Work out the finished part from the listing and answer in its coordinate system (mm). Face numbers are marked on the shaded views. A direction names the side the tool comes from. Coordinates: 2 decimals unless noted, no trailing zeros. Order: outer loops, then holes, each group sorted by start corner. A loop starts at its lowest first (then second) coordinate and runs counter-clockwise, first axis right, second up. Notation, with made-up numbers: (-8, 85) -> (1, 85) arc R4 ccw to (1, 91) -> close; hole circle Ø7 at (-15, -35). An arc over 180 degrees is marked (long way). Use one line per item in the form item = value.
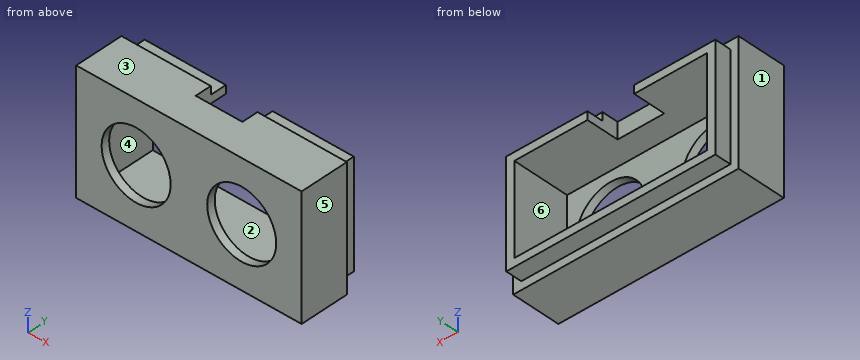
from build123d import *

# Parameters (mm, degrees)
SKETCH1_W           = 47.5
SKETCH1_H           = 22
SKETCH1_R           = 8.5
BOSS_EXTRUDE1_DEPTH = 2
SKETCH1_3_W         = 51.5
SKETCH1_3_H         = 26
SKETCH1_3_W_2       = 47.5
SKETCH1_3_H_2       = 22
BOSS_EXTRUDE2_DEPTH = 16
SKETCH1_5_W         = 55.5
SKETCH1_5_H         = 30
SKETCH1_5_W_2       = 51.5
SKETCH1_5_H_2       = 26
BOSS_EXTRUDE3_DEPTH = 12
SKETCH2_W           = 11.5
SKETCH2_H           = 8
CUT_EXTRUDE1_DEPTH  = 12


with BuildPart() as part:
    # Sketch1 → Boss-Extrude1 (new body)
    with BuildSketch(Plane(origin=(0, 0, 0), x_dir=(1, 0, 0), z_dir=(0, 1, 0))):
        Rectangle(SKETCH1_W, SKETCH1_H)
        with Locations(Location((-13, 0, 0), (0, 0, 270))):
            Circle(SKETCH1_R, mode=Mode.SUBTRACT)
        with Locations(Location((13, 0, 0), (0, 0, 270))):
            Circle(SKETCH1_R, mode=Mode.SUBTRACT)
    extrude(amount=BOSS_EXTRUDE1_DEPTH)

    # Sketch1_3 → Boss-Extrude2 (add)
    with BuildSketch(Plane(origin=(0, 0, 0), x_dir=(1, 0, 0), z_dir=(0, 1, 0))):
        Rectangle(SKETCH1_3_W, SKETCH1_3_H)
        Rectangle(SKETCH1_3_W_2, SKETCH1_3_H_2, mode=Mode.SUBTRACT)
    extrude(amount=BOSS_EXTRUDE2_DEPTH)

    # Sketch1_5 → Boss-Extrude3 (add)
    with BuildSketch(Plane(origin=(0, 0, 0), x_dir=(1, 0, 0), z_dir=(0, 1, 0))):
        Rectangle(SKETCH1_5_W, SKETCH1_5_H)
        Rectangle(SKETCH1_5_W_2, SKETCH1_5_H_2, mode=Mode.SUBTRACT)
    extrude(amount=BOSS_EXTRUDE3_DEPTH)

    # Sketch2 → Cut-Extrude1 (cut)
    with BuildSketch(Plane.XY.offset(15)):
        with Locations((0, 12)):
            Rectangle(SKETCH2_W, SKETCH2_H)
    extrude(amount=-CUT_EXTRUDE1_DEPTH, mode=Mode.SUBTRACT)


solid = part.part
(1) Section D-D on y = 14.25 is taken. Write down the section's boundary in (x, z), plus the area to 3 significant figures.
Data:
outline = (-25.75, -13) -> (25.75, -13) -> (25.75, 13) -> (5.75, 13) -> (5.75, 11) -> (23.75, 11) -> (23.75, -11) -> (-23.75, -11) -> (-23.75, 11) -> (-5.75, 11) -> (-5.75, 13) -> (-25.75, 13) -> close
area = 271 mm²
(2) Section C-C on x = -13 is taken. Write down the section's boundary in (y, z).
Data:
outline = (0, -15) -> (12, -15) -> (12, -13) -> (16, -13) -> (16, -11) -> (2, -11) -> (2, -8.5) -> (0, -8.5) -> close; (0, 8.5) -> (2, 8.5) -> (2, 11) -> (16, 11) -> (16, 13) -> (12, 13) -> (12, 15) -> (0, 15) -> close
(3) Section A-A on y = 7 is taken. Write down the section's boundary in (x, z), plus the area to 3 significant figures.
Data:
outline = (-27.75, -15) -> (27.75, -15) -> (27.75, 15) -> (-27.75, 15) -> close; hole (-23.75, -11) -> (23.75, -11) -> (23.75, 11) -> (-23.75, 11) -> close
area = 620 mm²
(4) Each of these flat-tipped pins is pushed along its axis until it touches: P1, Ø1.2, axis at x = 0.5, z = 13.5, coming from the +Y side; P2, Ø15, axis at x = -3.5, z = 2.5, coming from the +Y side; P3, Ø1.2, axis at y = 14.5, z = -2.5, coming from the +X side. Where does it stop, or does it pass through?
Data:
P1 = 8
P2 = 2
P3 = 25.75
(5) The mould has two halves that part along Z. Classify the marked faces 1, 2, 3 and 4: released by +Z, released by -Z, zero draft, split by the parting line, or undercut.
Data:
face_1 = zero draft
face_2 = undercut
face_3 = released by +Z
face_4 = undercut
(6) Which of the six approach directions +Z, -Z, +X, -X, +Y, -Y give full straight-line access (tool end or side, diameter ignored) to the marked faces 5 and 6?
Data:
face_5 = +Z, -Z, +X, +Y, -Y
face_6 = +Y
(7) Straight lines are drawn through the part: line 1 along X through (y, z) = (0.9, 0); line 2 along X through (y, z) = (2.75, 8.5); line 3 along X through (y, z) = (14.75, -5.25). For each, find the intervals that lie inside material, in ascending order.
Data:
line_1 = -27.75 to -21.5, -4.5 to 4.5, 21.5 to 27.75
line_2 = -27.75 to -23.75, 23.75 to 27.75
line_3 = -25.75 to -23.75, 23.75 to 25.75
(8) Section B-B on z = 5.75 is taken. Write down the section's boundary in (x, y), plus the area to 3 significant figures.
Data:
outline = (-27.75, 0) -> (-19.26, 0) -> (-19.26, 2) -> (-23.75, 2) -> (-23.75, 16) -> (-25.75, 16) -> (-25.75, 12) -> (-27.75, 12) -> close; (-6.74, 0) -> (6.74, 0) -> (6.74, 2) -> (-6.74, 2) -> close; (19.26, 0) -> (27.75, 0) -> (27.75, 12) -> (25.75, 12) -> (25.75, 16) -> (23.75, 16) -> (23.75, 2) -> (19.26, 2) -> close
area = 157 mm²
